from build123d import *

# Parameters (mm, degrees)
SALIENTE_EXTRUIR3_DEPTH = 16
CROQUIS6_R              = 5.5
CORTAR_EXTRUIR3_DEPTH   = 17
CORTAR_EXTRUIR4_DEPTH   = 83
CROQUIS8_W              = 18
CROQUIS8_H              = 4
CROQUIS8_W_2            = 12
CORTAR_EXTRUIR5_DEPTH   = 83
CROQUIS9_W              = 8
CROQUIS9_H              = 4
CORTAR_EXTRUIR6_DEPTH   = 83
CROQUIS10_W             = 7
CROQUIS10_H             = 4
SALIENTE_EXTRUIR4_DEPTH = 82
CROQUIS11_W             = 7
CROQUIS11_H             = 4
SALIENTE_EXTRUIR5_DEPTH = 82


with BuildPart() as part:
    # Croquis1 → Saliente-Extruir3 (new body)
    with BuildSketch(Plane(origin=(0, 0, 0), x_dir=(1, 0, 0), z_dir=(0, 1, 0))):
        with BuildLine():
            Line((-29, 68), (29, 68))
            ThreePointArc((29, 68), (37.485281374, 64.485281374), (41, 56))
            Line((41, 56), (41, -56))
            ThreePointArc((41, -56), (37.485281374, -64.485281374), (29, -68))
            Line((29, -68), (-29, -68))
            ThreePointArc((-29, -68), (-37.485281374, -64.485281374), (-41, -56))
            Line((-41, -56), (-41, 56))
            ThreePointArc((-41, 56), (-37.485281374, 64.485281374), (-29, 68))
        make_face()
    extrude(amount=SALIENTE_EXTRUIR3_DEPTH)

    # Croquis6 → Cortar-Extruir3 (cut, through all)
    with BuildSketch(Plane(origin=(0, 16, 0), x_dir=(1, 0, 0), z_dir=(0, 1, 0))):
        with Locations((-29, 56)):
            Circle(CROQUIS6_R)
        with Locations((29, 56)):
            Circle(CROQUIS6_R)
        with Locations((-29, -56)):
            Circle(CROQUIS6_R)
        with Locations((29, -56)):
            Circle(CROQUIS6_R)
    extrude(amount=-CORTAR_EXTRUIR3_DEPTH, mode=Mode.SUBTRACT)

    # Croquis7 → Cortar-Extruir4 (cut, through all)
    with BuildSketch(Plane.ZY.offset(41)):
        Polygon((0, 16), (-38, 16), (-38, 12), (38, 12), (38, 16), align=None)
    extrude(amount=-CORTAR_EXTRUIR4_DEPTH, mode=Mode.SUBTRACT)

    # Croquis8 → Cortar-Extruir5 (cut, through all)
    with BuildSketch(Plane.ZY.offset(41)):
        with Locations((-47, 2)):
            Rectangle(CROQUIS8_W, CROQUIS8_H)
        with Locations((-62, 2)):
            Rectangle(CROQUIS8_W_2, CROQUIS8_H)
        with Locations((47, 2)):
            Rectangle(CROQUIS8_W, CROQUIS8_H)
        with Locations((62, 2)):
            Rectangle(CROQUIS8_W_2, CROQUIS8_H)
    extrude(amount=-CORTAR_EXTRUIR5_DEPTH, mode=Mode.SUBTRACT)

    # Croquis9 → Cortar-Extruir6 (cut, through all)
    with BuildSketch(Plane.ZY.offset(41)):
        with Locations((34, 2)):
            Rectangle(CROQUIS9_W, CROQUIS9_H)
        with Locations((-34, 2)):
            Rectangle(CROQUIS9_W, CROQUIS9_H)
    extrude(amount=-CORTAR_EXTRUIR6_DEPTH, mode=Mode.SUBTRACT)

    # Croquis10 → Saliente-Extruir4 (add)
    with BuildSketch(Plane.ZY.offset(41)):
        with Locations((-34.5, 14)):
            Rectangle(CROQUIS10_W, CROQUIS10_H)
        with Locations((34.5, 14)):
            Rectangle(CROQUIS10_W, CROQUIS10_H)
    extrude(amount=-SALIENTE_EXTRUIR4_DEPTH)

    # Croquis11 → Saliente-Extruir5 (add)
    with BuildSketch(Plane.ZY.offset(41)):
        with Locations((-27.5, 14)):
            Rectangle(CROQUIS11_W, CROQUIS11_H)
        with Locations((27.5, 14)):
            Rectangle(CROQUIS11_W, CROQUIS11_H)
    extrude(amount=-SALIENTE_EXTRUIR5_DEPTH)


solid = part.part
For this review, take the finished solid that the model builds, in its own axes (mm). A direction names the side the tool comes from. Coordinates: 2 decimals unless noted, no trailing zeros. Write each loop counter-clockwise with the first axis right and the second up, starting at its lowest first coordinate (ties: lowest second). Pieces come first, ordered by that corner, then holes. Notation, with made-up numbers: (-30.75, -21) -> (7.25, -21) arc R23 ccw to (7.25, 5) -> close; hole circle Ø1 at (83, 60.5). An arc over 180 degrees is marked (long way). Write each question's results on one line, items separated by ' | '. Start each with the question number.
1) Consider section A-A (y = 14). Write out the cut boundary in (x, z), plus the area to 3 significant figures.
2) Wall thickness on L1, parallel to Z at x = 29, y = 11; L2, parallel to X at y = 9.75, z = -56; L3, parallel to X at y = 14.75, z = -52: over which ranges is each line inside the solid? List them lowest first. Write a range as [from, to].
3) The part is to be moulded in two halves that separate along X. For faces 6 (the face through (37.39, 9.92, -64.58)), 7 (the face through (-34.495, 10.084, 55.758)), 8 (the face through (-37.39, 9.92, 64.58)), 9 (the face through (-1, 12, 0)), say which applies: +X half, -X half, draft (parallel to the pull), parting line (faces both ways), or undercut.
4) For faces 1 (the face through (-1, 14, 24)), 2 (the face through (24.95, 10.08, -59.72)), 3 (the face through (-1, 2, 30)), 4 (the face through (-1, 2, -30)), 5 (the face through (37.58, 9.92, 64.39)), list the 3-axis set-ups (+Z, -Z, +X, -X, +Y, -Y) from which the entire face can be reached by the end or side of a thin tool; tool diameter is ignored.
5) Consider section B-B (y = 6.25). Write out the cut boundary in (x, z).
6) Insertion check: pin 1 (3 mm diameter, centred on x = 17, y = 3, fed in from +Z); pin 2 (10 mm diameter, centred on x = 29, z = 56, fed in from +Y); pin 3 (2 mm diameter, centred on x = 20.5, y = 2, fed in from -Z); pin 4 (2 mm diameter, centred on x = -19.5, z = -21, fed in from +Y). Each pin has a flat end and moves straight along its axis. Give the tip position at first contact, or say it passes through.
7) Consider section D-D (x = 8). Write out the cut boundary in (y, z), plus the area to 3 significant figures.
8) Consider section C-C (x = 27.5). Write out the cut boundary in (y, z), plus the area to 3 significant figures.
Geometry says:
1) outline: (-41, -56) arc R12 ccw to (-29, -68) -> (29, -68) arc R12 ccw to (41, -56) -> (41, -24) -> (-41, -24) -> close; (-41, 24) -> (41, 24) -> (41, 56) arc R12 ccw to (29, 68) -> (-29, 68) arc R12 ccw to (-41, 56) -> close; hole circle Ø11 at (-29, -56); hole circle Ø11 at (-29, 56); hole circle Ø11 at (29, -56); hole circle Ø11 at (29, 56) | area: 6,710 mm^2
2) L1: [-68, -61.5], [-50.5, 50.5], [61.5, 68] | L2: [-41, -34.5], [-23.5, 23.5], [34.5, 41] | L3: [-41, -32.77], [-25.23, 25.23], [32.77, 41]
3) face 6: +X half | face 7: undercut | face 8: -X half | face 9: draft
4) face 1: +X, -X, +Y | face 2: +Y, -Y | face 3: +Z, +X, -X, -Y | face 4: -Z, +X, -X, -Y | face 5: +Z, +X, +Y, -Y
5) outline: (-41, -56) arc R12 ccw to (-29, -68) -> (29, -68) arc R12 ccw to (41, -56) -> (41, 56) arc R12 ccw to (29, 68) -> (-29, 68) arc R12 ccw to (-41, 56) -> close; hole circle Ø11 at (-29, -56); hole circle Ø11 at (-29, 56); hole circle Ø11 at (29, -56); hole circle Ø11 at (29, 56)
6) pin 1: z = 68 | pin 2: through | pin 3: z = -30 | pin 4: y = 12
7) outline: (0, -30) -> (4, -30) -> (4, -68) -> (16, -68) -> (16, -24) -> (12, -24) -> (12, 24) -> (16, 24) -> (16, 68) -> (4, 68) -> (4, 30) -> (0, 30) -> close | area: 1,680 mm^2
8) outline: (0, -30) -> (4, -30) -> (4, -50.71) -> (16, -50.71) -> (16, -24) -> (12, -24) -> (12, 24) -> (16, 24) -> (16, 50.71) -> (4, 50.71) -> (4, 30) -> (0, 30) -> close; (4, -68) -> (16, -68) -> (16, -61.29) -> (4, -61.29) -> close; (4, 61.29) -> (16, 61.29) -> (16, 68) -> (4, 68) -> close | area: 1,430 mm^2
